For this review, use the dimensioned drawing (mm, ordinates from the lowest corner) and the shaded views. Round coordinates to 2 decimals unless told otherwise and drop trailing zeros. Loops run counter-clockwise (first coordinate to the right, second up) from the corner with the lowest first, then second, coordinate; pieces in that order, holes last. Notation, with made-up numbers: (32.5, -11) -> (43.5, -11) arc R18 ccw to (43.5, 20) -> close; hole circle Ø9 at (16.5, 44.5). An arc over 180 degrees is marked (long way). Answer as CSV lines item,"result". Start each with the question number.
(1) For P1, Ø4, axis at x = 7, y = 8.08, coming from the -Z side, flat-tipped, find the tip position at first contact; note if it passes through.
(2) To check wall thickness, follow line 1 (Y direction, x = 8.5, z = 5.5) (1 decimal); line 2 (X direction, y = 6.75, z = 4.25); line 3 (X direction, y = 7.25, z = 1.75). State the ranges of each line that lie inside material, in increasing order. Write a range as from..to.
(3) Draft analysis for pull direction Y (two halves, no side actions). For the marked faces 1, 2, 3 and 4, state which applies: +Y half, -Y half, draft (parallel to the pull), parting line (faces both ways), or undercut.
(4) Take a section at A-A, the plane z = 2. Write out the cut boundary in (x, y) (1 decimal).
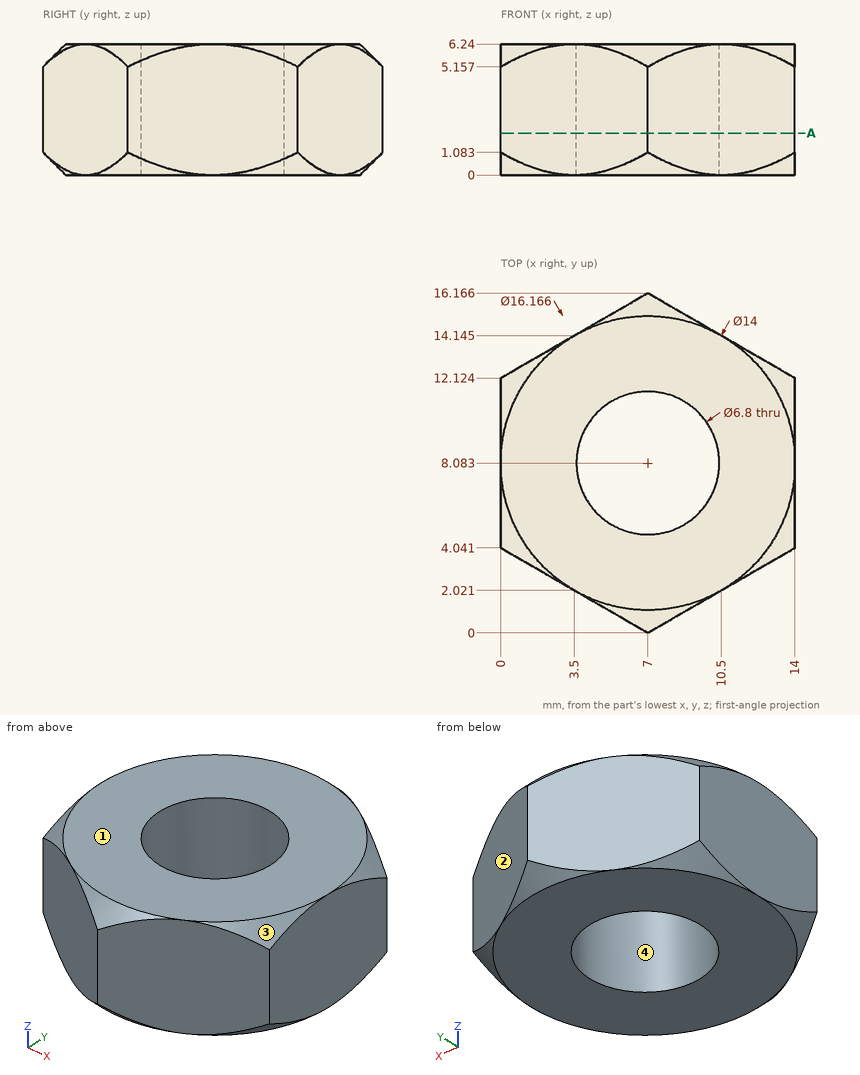
The answers:
1,P1,"through"
2,line 1,"0.9..5, 11.1..15.3"
2,line 2,"0..3.87, 10.13..14"
2,line 3,"0..3.7, 10.3..14"
3,face 1,"draft"
3,face 2,"+Y half"
3,face 3,"-Y half"
3,face 4,"undercut"
4,outline,"(0, 4) -> (7, 0) -> (14, 4) -> (14, 12.1) -> (7, 16.2) -> (0, 12.1) -> close; hole circle Ø6.8 at (7, 8.1)"
